Source: CAD feature listing. Evaluate the final solid. Frame: model axes, mm. A direction names the side the tool comes from. Coordinates: 2 decimals unless noted, no trailing zeros. Write each loop counter-clockwise with the first axis right and the second up, starting at its lowest first coordinate (ties: lowest second). Pieces come first, ordered by that corner, then holes. Notation, with made-up numbers: (21.25, 33) -> (54.25, 33) arc R30 cw to (54.25, 68) -> close; hole circle Ø8 at (77, 72). An arc over 180 degrees is marked (long way). Write item = value, one per line.
from build123d import *

# Parameters (mm, degrees)
SKETCH_1_R          = 15
EXTRUDE_1_DEPTH     = 40
EXTRUDE_2_DEPTH     = 8
SKETCH_3_R          = 6
CUT_EXTRUDE_1_DEPTH = 96
SKETCH_4_R          = 4
CUT_EXTRUDE_2_DEPTH = 96


with BuildPart() as part:
    # 草图1 → 凸台-拉伸1 (new body)
    with BuildSketch(Plane(origin=(0, -20, 0), x_dir=(1, 0, 0), z_dir=(0, 1, 0))):
        with Locations(Location((0, 0, 0), (0, 0, 270))):
            Circle(SKETCH_1_R)
    extrude(amount=EXTRUDE_1_DEPTH)

    # 草图2 → 凸台-拉伸2 (add)
    with BuildSketch(Plane(origin=(0, -20, 0), x_dir=(1, 0, 0), z_dir=(0, 1, 0))):
        with BuildLine():
            Line((1.071428571, 14.961685761), (70.714285714, 9.974457174))
            ThreePointArc((70.714285714, 9.974457174), (80, 0), (70.714285714, -9.974457174))
            Line((70.714285714, -9.974457174), (1.071428571, -14.961685761))
            ThreePointArc((1.071428571, -14.961685761), (-15, 0), (1.071428571, 14.961685761))
        make_face()
    extrude_2 = extrude(amount=EXTRUDE_2_DEPTH)

    # 镜向1: 凸台-拉伸2 across plane
    add(extrude_2.mirror(Plane.ZX))

    # 草图3 → 切除-拉伸1 (cut, symmetric)
    with BuildSketch(Plane(origin=(0, 0, 0), x_dir=(1, 0, 0), z_dir=(0, 1, 0))):
        with Locations(Location((0, 0, 0), (0, 0, 270))):
            Circle(SKETCH_3_R)
    extrude(amount=CUT_EXTRUDE_1_DEPTH, both=True, mode=Mode.SUBTRACT)

    # 草图4 → 切除-拉伸2 (cut, symmetric)
    with BuildSketch(Plane(origin=(0, 0, 0), x_dir=(1, 0, 0), z_dir=(0, 1, 0))):
        with Locations(Location((70, 0, 0), (0, 0, 270))):
            Circle(SKETCH_4_R)
    extrude(amount=CUT_EXTRUDE_2_DEPTH, both=True, mode=Mode.SUBTRACT)


solid = part.part
1) First-contact query: pin 1 Ø10 at (x, y) = (13.5, 1.5) entering from -Z; pin 2 Ø6 at (y, z) = (13.5, 10.5) entering from -X; pin 3 Ø1.5 at (y, z) = (0.5, 8.5) entering from -X; pin 4 Ø9 at (x, z) = (70, 0) entering from +Y. Flat tips, straight axial feed; report the tip coordinate or a pass-through.
Answer block:
pin_1 = -12.36
pin_2 = -12.99
pin_3 = -12.84
pin_4 = 20
2) Pull-direction query (X, two-part tool) for faces 3 (the flat face through (33, 20, 0)), 4 (the flat face through (35.405, 16.056, -12.503)), 5 (the cylindrical face through (66.095, -15.944, -0.867)); classes: +X half, -X half, draft (parallel to the pull), parting line (faces both ways), or undercut.
Answer block:
face_3 = draft
face_4 = +X half
face_5 = undercut
3) Reachability of faces 1 (the flat face through (33, -20, 0)), 2 (the cylindrical face through (-14.643, -0.28, -3.252)) from +Z, -Z, +X, -X, +Y, -Y: full face, straight path, thin tool, end or side. Return the list, or none.
Answer block:
face_1 = +Z, -Z, +X, -X, -Y
face_2 = none
4) Material intervals for probe 1 along X at (y, z) = (-17.75, 0); probe 2 along Y at (x, z) = (27.5, 12.5); probe 3 along X at (y, z) = (-5.5, -9), sorted ascending. Write a range as [from, to].
Answer block:
probe_1 = [-15, -6], [6, 66], [74, 80]
probe_2 = [-20, -12], [12, 20]
probe_3 = [-12, 12]
5) Cut plane D-D, the plane x = 41. Output: boundary loops of the cut face in (y, z).
Answer block:
outline = (-20, -12.1) -> (-12, -12.1) -> (-12, 12.1) -> (-20, 12.1) -> close; (12, -12.1) -> (20, -12.1) -> (20, 12.1) -> (12, 12.1) -> close
6) Cut plane B-B, the plane y = -15. Output: boundary loops of the cut face in (x, z).
Answer block:
outline = (1.07, -14.96) -> (70.71, -9.97) arc R10 ccw to (70.71, 9.97) -> (1.07, 14.96) arc R15 ccw (long way) to start; hole circle Ø12 at (0, 0); hole circle Ø8 at (70, 0)
7) Cut plane C-C, the plane z = 0. Output: boundary loops of the cut face in (x, y), and give its area (3 significant figures).
Answer block:
outline = (-15, -20) -> (-6, -20) -> (-6, 20) -> (-15, 20) -> close; (6, -20) -> (66, -20) -> (66, -12) -> (15, -12) -> (15, 12) -> (66, 12) -> (66, 20) -> (6, 20) -> close; (74, -20) -> (80, -20) -> (80, -12) -> (74, -12) -> close; (74, 12) -> (80, 12) -> (80, 20) -> (74, 20) -> close
area = 1,630 mm2
8) Cut plane A-A, the plane x = 0. Output: boundary loops of the cut face in (y, z).
Answer block:
outline = (-20, -15) -> (20, -15) -> (20, -6) -> (-20, -6) -> close; (-20, 6) -> (20, 6) -> (20, 15) -> (-20, 15) -> close
